from build123d import *

# Parameters (mm, degrees)
F1_DEPTH  = 13.8
F2_W      = 5.4
F2_H      = 40
F3_DEPTH  = 17
F4_R      = 3
F5_DEPTH  = 25
F6_R      = 3
F7_DEPTH  = 6
F8_R      = 4.5
F9_DEPTH  = 2.5
F10_R     = 4
F11_W     = 10
F11_H     = 40
F12_DEPTH = 20
F13_R     = 7.5
F14_DEPTH = 4.7
F15_R     = 7.5
F16_DEPTH = 4.7
F17_R     = 1.9
F18_DEPTH = 70


with BuildPart() as f1:
    # F0 (on Front) → F1 (new body)
    with BuildSketch(Plane.XZ):
        Polygon((11.3874197267, 30.6198454252), (-3.6125802733, 30.6198454252), (-3.6125802733, -9.3801545748), (11.3874197267, -9.3801545748), (16.3874197267, -9.3801545748), (16.3874197267, 5.6198454252), (16.3874197267, 25.6198454252), (16.3874197267, 30.6198454252), align=None)
    extrude(amount=F1_DEPTH)

    # F2 (on face) → F3 (cut)
    with BuildSketch(Plane(origin=(-3.6125802733, 0, 0), x_dir=(0, -1, 0), z_dir=(-1, 0, 0))):
        with Locations((6.9, 10.6198454252)):
            Rectangle(F2_W, F2_H)
    extrude(amount=-F3_DEPTH, mode=Mode.SUBTRACT)

    # F4 (on face) → F5 (cut)
    with BuildSketch(Plane(origin=(0, 0, 0), x_dir=(-1, 0, 0), z_dir=(0, 1, 0))):
        with Locations((-7.1874197267, 25.6198454252)):
            Circle(F4_R)
        with Locations((-7.1874197267, -4.3801545748)):
            Circle(F4_R)
    extrude(amount=-F5_DEPTH, mode=Mode.SUBTRACT)

    # F6 (on face) → F7 (join)
    with BuildSketch(Plane.XZ):
        with Locations((0.9593699942, 19.8055244982)):
            Circle(F6_R)
    extrude(amount=-F7_DEPTH)

    # F8 (on face) → F9 (join)
    with BuildSketch(Plane(origin=(0, 6, 0), x_dir=(-1, 0, 0), z_dir=(0, 1, 0))):
        with Locations((-0.9593699942, 19.8055244982)):
            Circle(F8_R)
    extrude(amount=F9_DEPTH)

    # F10
    f10_edges = [f1.edges().sort_by_distance(p)[0] for p in [
        (-3.61258, -2.1, 30.619845),
        (-3.61258, -11.7, 30.619845),
        (-3.61258, -2.1, -9.380155),
        (-3.61258, -11.7, -9.380155),
    ]]
    fillet(f10_edges, radius=F10_R)

    # F11 (on face) → F12 (join)
    with BuildSketch(Plane.YZ.offset(16.3874197267)):
        with Locations((-6.9, 10.6198454252)):
            Rectangle(F11_W, F11_H)
    extrude(amount=F12_DEPTH)

    # F13 (on face) → F14 (join)
    with BuildSketch(Plane.XY.offset(30.6198454252)):
        with Locations((41.7828261852, -6.9)):
            Circle(F13_R)
    extrude(amount=-F14_DEPTH)

    # F15 (on face) → F16 (join)
    with BuildSketch(Plane(origin=(0, 0, -9.3801545748), x_dir=(1, 0, 0), z_dir=(0, 0, -1))):
        with Locations((41.7574755847, 6.4750881866)):
            Circle(F15_R)
    extrude(amount=-F16_DEPTH)

    # F17 (on face) → F18 (cut)
    with BuildSketch(Plane(origin=(0, 0, -9.3801545748), x_dir=(1, 0, 0), z_dir=(0, 0, -1))):
        with Locations((41.7574755847, 6.4750881866)):
            Circle(F17_R)
    extrude(amount=-F18_DEPTH, mode=Mode.SUBTRACT)


solid = f1.part
Geometry: final body of the model. Coordinates: model frame, mm. A direction names the side the tool comes from. Coordinates: 2 decimals unless noted, no trailing zeros. Loops run counter-clockwise (first coordinate to the right, second up) from the corner with the lowest first, then second, coordinate; pieces in that order, holes last. Notation, with made-up numbers: M -39.75,2 L -2.75,2 A9 ccw -2.75,9 Z; hole C 26.5,-8.75 d1. An arc over 180 degrees is marked long. One line per item, written item: value. Start each with the question number.
1) Cut plane C-C (z = 14). Return loops of the section in (x, y), then the cut area to 3 significant figures.
2) Material intervals for L1, parallel to Y at x = 5.5, z = 0.5; L2, parallel to Z at x = 44, y = -3.75; L3, parallel to Y at x = 18, z = 16, sorted ascending. Write a range as from..to.
3) Cut plane D-D (y = -7.5). Return loops of the section in (x, z), then the cut area to 3 significant figures.
4) Draft query along Y for faces 6 (the flat face through (36.387, -7, 9)), 7 (the flat face through (13.387, -7, 11)), 8 (the flat face through (6, -13.8, 11)). Return one class per face: released by +Y, released by -Y, zero draft, split by the parting line, or undercut.
5) Pin query (flat end, axial travel): P1, Ø3, axis at x = 9.5, z = 22, coming from the +Y side; P2, Ø8, axis at x = 7.19, z = 25.62, coming from the -Y side; P3, Ø1.5, axis at y = -5.5, z = 3, coming from the +X side. Return the tip coordinate at first contact, or that it passes through.
6) Reachability of faces 1 (the flat face through (5, -9.6, 10)), 2 (the flat face through (16.387, -13, 10)), 3 (the cylindrical face through (49.28, -7.15, 28.3)), 4 (the cylindrical face through (0.57, 2.96, 22.78)), 5 (the flat face through (42.6, -8.5, 25.92)) from +Z, -Z, +X, -X, +Y, -Y: full face, straight path, thin tool, end or side. Return the list, or none.
7) Cut plane A-A (x = 11.5). Return loops of the section in (y, z).
8) Cut plane B-B (y = -1). Return loops of the section in (x, z).
Evaluation:
1. outline: M -3.61,-13.8 L 16.39,-13.8 L 16.39,-11.9 L 36.39,-11.9 L 36.39,-1.9 L 16.39,-1.9 L 16.39,0 L -3.61,0 L -3.61,-4.2 L 13.39,-4.2 L 13.39,-9.6 L -3.61,-9.6 Z
1. area: 384 mm^2
2. L1: -13.8..-9.6, -4.2..0
2. L2: -9.38..-4.68, 25.92..30.62
2. L3: -11.9..-1.9
3. outline: M 13.39,-9.38 L 40.16,-9.38 L 40.16,-4.68 L 36.39,-4.68 L 36.39,25.92 L 40.16,25.92 L 40.16,30.62 L 13.39,30.62 Z; M 43.36,-9.38 L 49.19,-9.38 L 49.19,-4.68 L 43.36,-4.68 Z; M 43.36,25.92 L 49.26,25.92 L 49.26,30.62 L 43.36,30.62 Z
3. area: 1,010 mm^2
4. face 6: zero draft
4. face 7: undercut
4. face 8: released by -Y
5. P1: y = 0
5. P2: y = -13.8
5. P3: x = 36.39
6. face 1: +Z, -Z, -X
6. face 2: +Z, -Z, -Y
6. face 3: +Z
6. face 4: none
6. face 5: +X, +Y, -Y
7. outline: M -13.8,-9.38 L -9.6,-9.38 L -9.6,30.62 L -13.8,30.62 Z; M -4.2,-9.38 L 0,-9.38 L 0,30.62 L -4.2,30.62 Z
8. outline: M -3.61,-5.38 A4 ccw 0.39,-9.38 L 16.39,-9.38 L 16.39,30.62 L 0.39,30.62 A4 ccw -3.61,26.62 Z; M 36.63,-9.38 L 46.88,-9.38 L 46.88,-4.68 L 36.63,-4.68 Z; M 37.15,25.92 L 46.41,25.92 L 46.41,30.62 L 37.15,30.62 Z; hole C 7.19,-4.38 d6; hole C 7.19,25.62 d6
